Input: dimensioned drawing with shaded views. Units: mm. Origin: part minimum x, y, z. A direction names the side the tool comes from. Give positions to 0.01 mm unless a question says otherwise; leave off trailing zeros. Write each loop counter-clockwise with the first axis right and the second up, starting at its lowest first coordinate (ties: lowest second). Pieces come first, ordered by that corner, then holes. Notation, with made-up numbers: (-11, 89) -> (-3, 89) arc R17 cw to (-3, 110) -> close; hole circle Ø9 at (-20, 71). An arc over 180 degrees is marked (long way). Return JSON: item names as keys, results as strings. Group by question number.
Item 1: Line query: line 1 (X direction, y = 1.65, z = 5); line 2 (Z direction, x = 31.2, y = 0.95); line 3 (X direction, y = 7, z = 9.5). Output: solid intervals per line, ascending. Write a range as [from, to].
Item 2: Section D-D, the plane x = 5. Return loops of the section in (y, z).
Item 3: Section C-C, the plane y = 7.5. Return loops of the section in (x, z).
Item 4: Set-up query: the marked faces 1, 2, 3 and 4. Return all of +Z, -Z, +X, -X, +Y, -Y with unobstructed straight access to the full face (end or side cutting, diameter ignored); none if empty.
Item 5: Mould query, pull axis X, two halves, no side actions, for the marked faces 5, 6, 7 and 8. Classes: released by +X, released by -X, zero draft, split by the parting line, or undercut.
Item 6: Section B-B, the plane z = 5. Return loops of the section in (x, y).
Item 7: Section A-A, the plane y = 0.5. Return loops of the section in (x, z).
Item 8: Pin query (flat end, axial travel): P1, Ø6, axis at y = 7, z = 1.5, coming from the +X side; P2, Ø4.5, axis at y = 6, z = 3, coming from the -X side; P3, Ø5, axis at x = 31.2, z = 5, coming from the +Y side. Return the tip coordinate at first contact, or that it passes through.
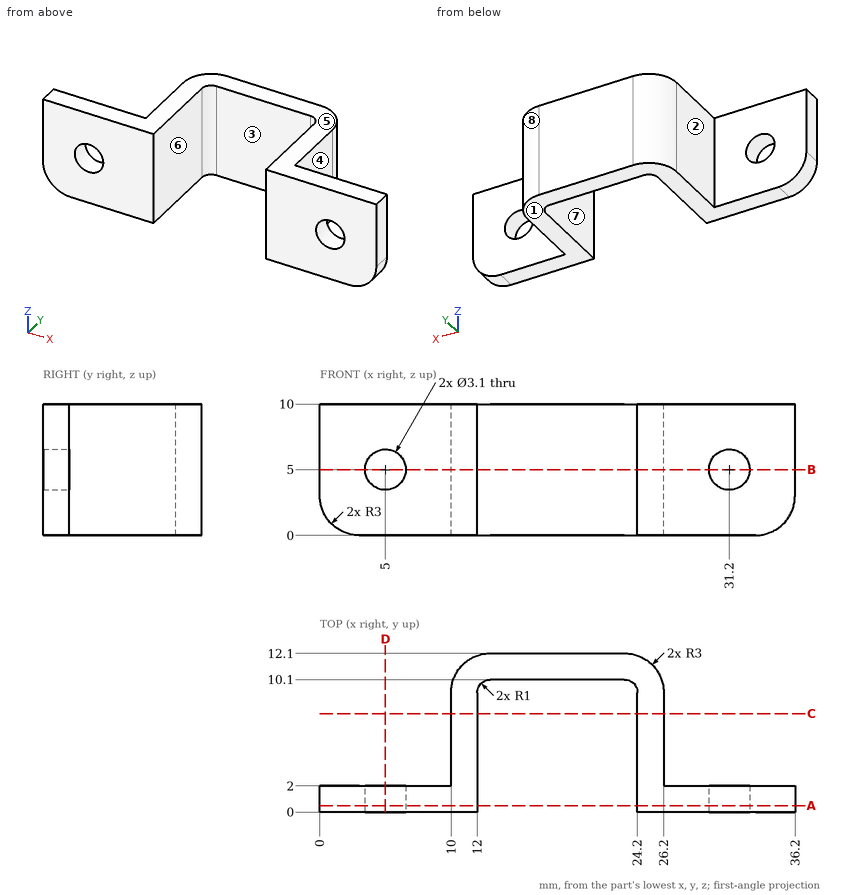
Answer below:
{
 "1": {"line 1": "x = [0, 3.45], [6.55, 12], [24.2, 29.65], [32.75, 36.2]", "line 2": "z = [0, 3.45], [6.55, 10]", "line 3": "x = [10, 12], [24.2, 26.2]"},
 "2": {"outline": "(0, 0) -> (2, 0) -> (2, 3.45) -> (0, 3.45) -> close; (0, 6.55) -> (2, 6.55) -> (2, 10) -> (0, 10) -> close"},
 "3": {"outline": "(10, 0) -> (12, 0) -> (12, 10) -> (10, 10) -> close; (24.2, 0) -> (26.2, 0) -> (26.2, 10) -> (24.2, 10) -> close"},
 "4": {"face 1": "-Z, +X, -X, +Y, -Y", "face 2": "+Z, -Z, -X, +Y", "face 3": "+Z, -Z, -Y", "face 4": "+Z, -Z, +X, +Y"},
 "5": {"face 5": "zero draft", "face 6": "undercut", "face 7": "undercut", "face 8": "released by +X"},
 "6": {"outline": "(0, 0) -> (3.45, 0) -> (3.45, 2) -> (0, 2) -> close; (6.55, 0) -> (12, 0) -> (12, 9.1) arc R1 cw to (13, 10.1) -> (23.2, 10.1) arc R1 cw to (24.2, 9.1) -> (24.2, 0) -> (29.65, 0) -> (29.65, 2) -> (26.2, 2) -> (26.2, 9.1) arc R3 ccw to (23.2, 12.1) -> (13, 12.1) arc R3 ccw to (10, 9.1) -> (10, 2) -> (6.55, 2) -> close; (32.75, 0) -> (36.2, 0) -> (36.2, 2) -> (32.75, 2) -> close"},
 "7": {"outline": "(0, 3) arc R3 ccw to (3, 0) -> (12, 0) -> (12, 10) -> (0, 10) -> close; (24.2, 0) -> (33.2, 0) arc R3 ccw to (36.2, 3) -> (36.2, 10) -> (24.2, 10) -> close; hole circle Ø3.1 at (5, 5); hole circle Ø3.1 at (31.2, 5)"},
 "8": {"P1": "stops at x = 26.2", "P2": "stops at x = 10", "P3": "stops at y = 2"}
}
